CAD build for the part. Positions are in the model's coordinates, mm. Face numbers are marked on the shaded views. Give positions to 0.01 mm unless a question says otherwise; leave off trailing zeros. Order: outer loops, then holes, each group sorted by start corner. A loop starts at its lowest first (then second) coordinate and runs counter-clockwise, first axis right, second up. Notation, with made-up numbers: M -37,-27.75 L -11,-27.75 A11 cw -11,-16.75 Z; hole C 0.25,10 d3. An arc over 180 degrees is marked long. Put each result on its own line as item: value. Start each with the question number.
1) Two-plate mould, pull along X, no slides. Class the marked faces 1, 2, 3 and 4: released by +X, released by -X, zero draft, split by the parting line, or undercut.
2) Cut at C-C (y = -25). Write the cut outline in (x, z) (3 decimals), and give its area (3 significant figures).
3) Cut at B-B (z = 2.5). Write the cut outline in (x, y), and give its area (3 significant figures).
4) Drill centre lines: line 1 (X direction, y = -25, z = -0.25); line 2 (X direction, y = -24, z = 3). Where is each one in solid material? Low to high. Write a range as [from, to].
5) Cut at A-A (x = 0). Write the cut outline in (y, z) (3 decimals).
```python
from build123d import *

# Parameters (mm, degrees)
SKETCH1_R           = 19.25
SKETCH1_R_2         = 2.65
BOSS_EXTRUDE1_DEPTH = 4.125


with BuildPart() as part:
    # Sketch1 → Boss-Extrude1 (new, symmetric)
    with BuildSketch(Plane.XY):
        with BuildLine():
            Line((30, -26), (30, 26))
            ThreePointArc((30, 26), (28.828427125, 28.828427125), (26, 30))
            Line((26, 30), (-26, 30))
            ThreePointArc((-26, 30), (-28.828427125, 28.828427125), (-30, 26))
            Line((-30, 26), (-30, -26))
            ThreePointArc((-30, -26), (-28.828427125, -28.828427125), (-26, -30))
            Line((-26, -30), (26, -30))
            ThreePointArc((26, -30), (28.828427125, -28.828427125), (30, -26))
        make_face()
        with Locations(Location((0, 0, 0), (0, 0, 180))):
            Circle(SKETCH1_R, mode=Mode.SUBTRACT)
        with Locations(Location((-25, -25, 0), (0, 0, 180))):
            Circle(SKETCH1_R_2, mode=Mode.SUBTRACT)
        with Locations(Location((-25, 25, 0), (0, 0, 180))):
            Circle(SKETCH1_R_2, mode=Mode.SUBTRACT)
        with Locations(Location((25, -25, 0), (0, 0, 180))):
            Circle(SKETCH1_R_2, mode=Mode.SUBTRACT)
        with Locations(Location((25, 25, 0), (0, 0, 180))):
            Circle(SKETCH1_R_2, mode=Mode.SUBTRACT)
    extrude(amount=BOSS_EXTRUDE1_DEPTH, both=True)


solid = part.part
```
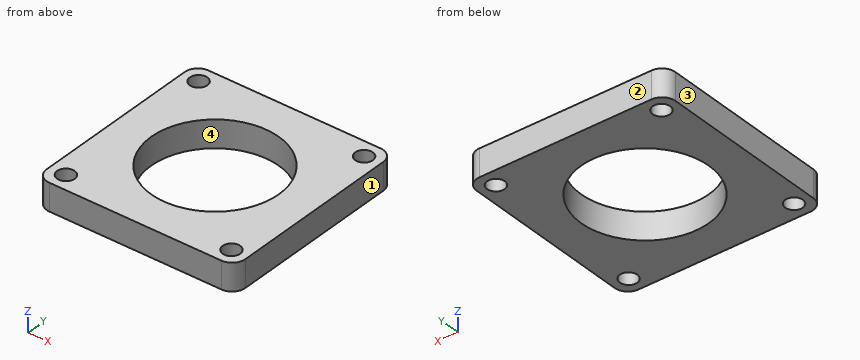
Solution:
1. face 1: released by +X
1. face 2: zero draft
1. face 3: released by -X
1. face 4: undercut
2. outline: M -30,-4.125 L -27.65,-4.125 L -27.65,4.125 L -30,4.125 Z; M -22.35,-4.125 L 22.35,-4.125 L 22.35,4.125 L -22.35,4.125 Z; M 27.65,-4.125 L 30,-4.125 L 30,4.125 L 27.65,4.125 Z
2. area: 408 mm²
3. outline: M -30,-26 A4 ccw -26,-30 L 26,-30 A4 ccw 30,-26 L 30,26 A4 ccw 26,30 L -26,30 A4 ccw -30,26 Z; hole C -25,-25 d5.3; hole C -25,25 d5.3; hole C 0,0 d38.5; hole C 25,-25 d5.3; hole C 25,25 d5.3
3. area: 2,330 mm²
4. line 1: [-30, -27.65], [-22.35, 22.35], [27.65, 30]
4. line 2: [-30, -27.45], [-22.55, 22.55], [27.45, 30]
5. outline: M -30,-4.125 L -19.25,-4.125 L -19.25,4.125 L -30,4.125 Z; M 19.25,-4.125 L 30,-4.125 L 30,4.125 L 19.25,4.125 Z
